For this review, take the finished solid that the model builds, in its own axes (mm). A direction names the side the tool comes from. Give positions to 0.01 mm unless a question says otherwise; leave off trailing zeros. Write each loop counter-clockwise with the first axis right and the second up, starting at its lowest first coordinate (ties: lowest second). Pieces come first, ordered by that corner, then holes. Notation, with made-up numbers: (-21, 49) -> (35, 49) arc R29 ccw to (35, 87) -> close; hole circle Ø4 at (-16, -15.5). An arc over 180 degrees is marked (long way). Return JSON: item names as keys, results as strings.
from build123d import *

# Parameters (mm, degrees)
F0_R     = 50
F1_DEPTH = 20
F2_R     = 32
F3_DEPTH = 25
F5_D     = 34


with BuildPart() as f1:
    # F0 (on Top) → F1 (new body)
    with BuildSketch(Plane.XY):
        with Locations((0, 1.086205)):
            Circle(F0_R)
    extrude(amount=F1_DEPTH)

    # F2 (on face) → F3 (join)
    with BuildSketch(Plane.XY.offset(20)):
        Circle(F2_R)
    extrude(amount=F3_DEPTH)

    # F5 (through all)
    with Locations(Plane.XY.offset(45)):
        with Locations((0, 0)):
            Hole(F5_D / 2)


solid = f1.part
1. The part is to be moulded in two halves that separate along X. For faces 3 (the flat face through (-12, 13, 0)), 4 (the cylindrical face through (-6.94, -31.24, 32.33)), 5 (the cylindrical face through (-9.139, 14.334, 22.185)), say which applies: +X half, -X half, draft (parallel to the pull), parting line (faces both ways), or undercut.
Results found:
{"face 3": "draft", "face 4": "parting line", "face 5": "undercut"}
2. Add section D-D, the plane z = 27. State the section outline as (x, y) points.
Results found:
{"outline": "circle Ø64 at (0, 0); hole circle Ø34 at (0, 0)"}
3. Add section C-C, the plane y = 26.5. State the section outline as (x, z) points.
Results found:
{"outline": "(-43.06, 0) -> (43.06, 0) -> (43.06, 20) -> (17.94, 20) -> (17.94, 45) -> (-17.94, 45) -> (-17.94, 20) -> (-43.06, 20) -> close"}
4. For pin 1 (12 mm diameter, centred on x = -32, z = 14, fed in from +Y); pin 2 (1.5 mm diameter, centred on x = 8, z = 30.5, fed in from +Y); pin 3 (6 mm diameter, centred on y = 2, z = 11.5, fed in from +X); pin 4 (1.5 mm diameter, centred on y = -4.5, z = 36.5, fed in from +X), all flat-tipped, find the tip position at first contact; note any pin that passes through.
Results found:
{"pin 1": "stops at y = 43.79", "pin 2": "stops at y = 31.17", "pin 3": "stops at x = 50", "pin 4": "stops at x = 31.78"}
5. For faces 1 (the flat face through (14, -14, 45)), 2 (the flat face through (22, 24, 20)), list the 3-axis set-ups (+Z, -Z, +X, -X, +Y, -Y) from which the entire face can be reached by the end or side of a thin tool; tool diameter is ignored.
Results found:
{"face 1": "+Z, +X, -X, +Y, -Y", "face 2": "+Z"}
6. Add section A-A, the plane x = 0. State the section outline as (y, z) points.
Results found:
{"outline": "(-48.91, 0) -> (-17, 0) -> (-17, 45) -> (-32, 45) -> (-32, 20) -> (-48.91, 20) -> close; (17, 0) -> (51.09, 0) -> (51.09, 20) -> (32, 20) -> (32, 45) -> (17, 45) -> close"}
7. Add section B-B, the plane y = 3.5. State the section outline as (x, z) points, plus the area to 3 significant figures.
Results found:
{"outline": "(-49.94, 0) -> (-16.64, 0) -> (-16.64, 45) -> (-31.81, 45) -> (-31.81, 20) -> (-49.94, 20) -> close; (16.64, 0) -> (49.94, 0) -> (49.94, 20) -> (31.81, 20) -> (31.81, 45) -> (16.64, 45) -> close", "area": "2,090 mm²"}
8. To check wall thickness, follow probe 1 along Y at (x, z) = (0, 17.5); probe 2 along Z at (x, y) = (-34.5, 5.5); probe 3 along Y at (x, z) = (5, 18.5). State the ranges of each line that lie inside material, in increasing order.
Results found:
{"probe 1": "y = -48.91 to -17, 17 to 51.09", "probe 2": "z = 0 to 20", "probe 3": "y = -48.66 to -16.25, 16.25 to 50.84"}
